from build123d import *

# Parameters (mm, degrees)
F0_R     = 25.336511
F1_DEPTH = 3.81
F2_T     = -2.54
F4_D     = 3.81
F4_DEPTH = 2.54


with BuildPart() as f1:
    # F0 (on Right) → F1 (new body)
    with BuildSketch(Plane.YZ):
        with Locations((0, -2.190114)):
            Circle(F0_R)
    extrude(amount=-F1_DEPTH)

    # F2
    f2_openings = [f1.faces().sort_by_distance(p)[0] for p in [
        (-3.81, 0, -2.190114),
    ]]
    offset(amount=F2_T, openings=f2_openings)

    # F4
    with Locations(Plane(origin=(-2.54, 0, 0), x_dir=(0, -1, 0), z_dir=(-1, 0, 0))):
        with Locations((0, 15.737751)):
            Hole(F4_D / 2, depth=F4_DEPTH)


solid = f1.part
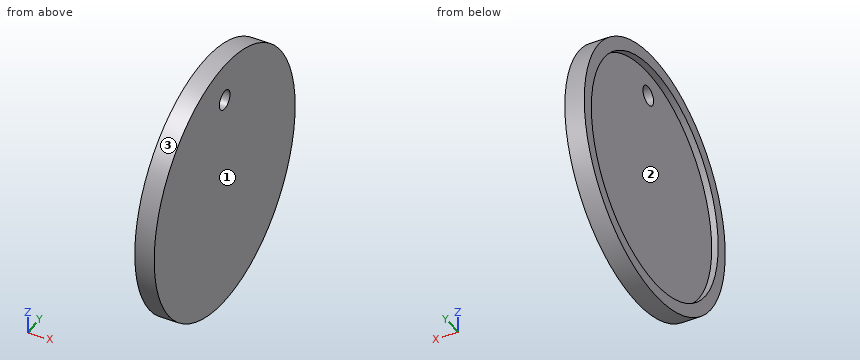
Can you work these out from the model? Positions are in its coordinate system, mm. Face numbers are marked on the shaded views. Give positions to 0.01 mm unless a question says otherwise; leave off trailing zeros. Write each loop counter-clockwise with the first axis right and the second up, starting at its lowest first coordinate (ties: lowest second). Pieces come first, ordered by that corner, then holes. Notation, with made-up numbers: M 4.5,-4.75 L 23.5,-4.75 A33 cw 23.5,34.25 Z; hole C 27.5,38 d5. An arc over 180 degrees is marked long. Answer in a Markdown table with one row per item. Add a question column.
Item 1: Please list where these lines run through material, in increasing order: L1, parallel to Z at x = -3.25, y = 0; L2, parallel to Z at x = -0.85, y = 0; L3, parallel to X at y = -21.5, z = 2.
Item 2: For pin 1 Ø4 at (y, z) = (7.5, 13) entering from -X; pin 2 Ø1.5 at (x, y) = (-3.5, 8.5) entering from -Z, each with a flat end and sliding along its axis, tell me the tip position at first contact or that it passes through.
Item 3: Imagine slicing it at D-D, the plane x = -1.7. Write out the boundary of the cut face in (y, z) (3 decimals), plus the area to 3 significant figures.
Item 4: Imagine slicing it at C-C, the plane y = 14.5. Write out the boundary of the cut face in (x, z).
Item 5: Imagine slicing it at B-B, the plane z = -21.5. Write out the boundary of the cut face in (x, y), plus the area to 3 significant figures.
Item 6: We'd pull the mould along Z, two halves only. Please class the marked faces 1, 2 and 3: released by +Z, released by -Z, zero draft, split by the parting line, or undercut.
Item 7: Imagine slicing it at A-A, the plane y = 0. Write out the boundary of the cut face in (x, z).
Evaluation:
| question | item | result |
|---|---|---|
| 1 | L1 | z = -27.53 to -24.99, 20.61 to 23.15 |
| 1 | L2 | z = -27.53 to 13.83, 17.64 to 23.15 |
| 1 | L3 | x = -2.54 to 0 |
| 2 | pin 1 | stops at x = -2.54 |
| 2 | pin 2 | stops at z = -26.31 |
| 3 | outline | C 0,-2.19 d50.673; hole C 0,15.738 d3.81 |
| 3 | area | 2,010 mm² |
| 4 | outline | M -3.81,-22.97 L 0,-22.97 L 0,18.59 L -3.81,18.59 L -3.81,15.4 L -2.54,15.4 L -2.54,-19.78 L -3.81,-19.78 Z |
| 5 | outline | M -3.81,-16.4 L 0,-16.4 L 0,16.4 L -3.81,16.4 L -3.81,12.12 L -2.54,12.12 L -2.54,-12.12 L -3.81,-12.12 Z |
| 5 | area | 94.2 mm² |
| 6 | face 1 | zero draft |
| 6 | face 2 | undercut |
| 6 | face 3 | split by the parting line |
| 7 | outline | M -3.81,-27.53 L 0,-27.53 L 0,13.83 L -2.54,13.83 L -2.54,-24.99 L -3.81,-24.99 Z; M -3.81,20.61 L -2.54,20.61 L -2.54,17.64 L 0,17.64 L 0,23.15 L -3.81,23.15 Z |
